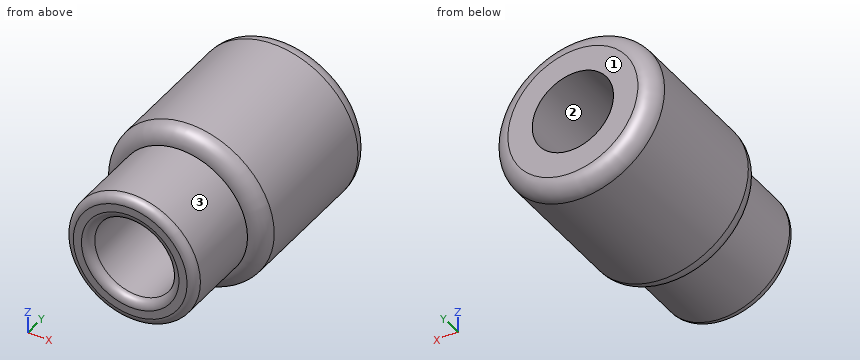
```python
from build123d import *

# Parameters (mm, degrees)
F0_R     = 127
F1_DEPTH = 254
F2_R     = 25.4
F4_D     = 127
F5_DEPTH = 127
F6_R     = 12.7


# Not quite as in the source:
# - a feature names something its author has since deleted; it is built from what else it names


with BuildPart() as f1:
    # F0 (on Front) → F1 (new body)
    with BuildSketch(Plane.XZ):
        Circle(F0_R)
    extrude(amount=F1_DEPTH)

    # F2
    f2_edges = [f1.edges().sort_by_distance(p)[0] for p in [
        (-127, -254, 0),
        (-127, 0, 0),
    ]]
    fillet(f2_edges, radius=F2_R)

    # F4 (through all)
    with Locations(Plane.XZ.offset(254)):
        with Locations((0, 0)):
            Hole(F4_D / 2)

    # F5 (add): a face of the model
    f5_faces = [f1.faces().sort_by_distance(p)[0] for p in [
        (-98.7263180413, -254, 0),
    ]]
    extrude(f5_faces, amount=F5_DEPTH)

    # F6
    f6_edges = [f1.edges().sort_by_distance(p)[0] for p in [
        (-101.6, -381, 0),
        (-63.5, -381, 0),
    ]]
    fillet(f6_edges, radius=F6_R)


solid = f1.part
```
Model file for the job. Use its own axes, mm. Face numbers are marked on the shaded views. Coordinates: 2 decimals unless noted, no trailing zeros. Order: outer loops, then holes, each group sorted by start corner. A loop starts at its lowest first (then second) coordinate and runs counter-clockwise, first axis right, second up. Notation, with made-up numbers: (42, 68) -> (80, 68) arc R17 ccw to (80, 79) -> close; hole circle Ø5 at (11, 67.5). An arc over 180 degrees is marked (long way). Answer as a JSON object with one key per item and string values. Group by question number.
1) Flat gauge pins, fed straight in: pin 1 (2 mm diameter, centred on y = -223.5, z = 40.5, fed in from -X); pin 2 (8 mm diameter, centred on x = -94.5, y = -201.5, fed in from +Z); pin 3 (1 mm diameter, centred on x = -45, y = -309.5, fed in from +Z). Where does each tip first touch, or does it go through?
2) Cut at A-A, the plane x = 0. Write the cut outline in (y, z).
3) Cut at B-B, the plane z = 0. Write the cut outline in (x, y).
4) Pull direction Z, two halves, no side cores. Call the marked faces 1, 2 and 3: +Z half, -Z half, draft (parallel to the pull), parting line (faces both ways), or undercut.
5) Cut at C-C, the plane y = -205. Write the cut outline in (x, z).
6) Drill centre lines: L1, parallel to Z at x = 0, y = -214; L2, parallel to Z at x = 0, y = -288; L3, parallel to X at y = -274, z = 22. Where is each one in solid material? Low to high.
Check values:
{
 "1": {"pin 1": "stops at x = -120.7", "pin 2": "stops at z = 89.1", "pin 3": "stops at z = 91.34"},
 "2": {"outline": "(-381, -88.9) arc R12.7 ccw to (-368.3, -101.6) -> (-254, -101.6) arc R25.4 ccw to (-228.6, -127) -> (-25.4, -127) arc R25.4 ccw to (0, -101.6) -> (0, -63.5) -> (-368.3, -63.5) arc R12.7 ccw to (-381, -76.2) -> close; (-381, 76.2) arc R12.7 ccw to (-368.3, 63.5) -> (0, 63.5) -> (0, 101.6) arc R25.4 ccw to (-25.4, 127) -> (-228.6, 127) arc R25.4 ccw to (-254, 101.6) -> (-368.3, 101.6) arc R12.7 ccw to (-381, 88.9) -> close"},
 "3": {"outline": "(-127, -228.6) arc R25.4 ccw to (-101.6, -254) -> (-101.6, -368.3) arc R12.7 ccw to (-88.9, -381) -> (-76.2, -381) arc R12.7 ccw to (-63.5, -368.3) -> (-63.5, 0) -> (-101.6, 0) arc R25.4 ccw to (-127, -25.4) -> close; (63.5, -368.3) arc R12.7 ccw to (76.2, -381) -> (88.9, -381) arc R12.7 ccw to (101.6, -368.3) -> (101.6, -254) arc R25.4 ccw to (127, -228.6) -> (127, -25.4) arc R25.4 ccw to (101.6, 0) -> (63.5, 0) -> close"},
 "4": {"face 1": "draft", "face 2": "undercut", "face 3": "parting line"},
 "5": {"outline": "circle Ø254 at (0, 0); hole circle Ø127 at (0, 0)"},
 "6": {"L1": "z = -127 to -63.5, 63.5 to 127", "L2": "z = -101.6 to -63.5, 63.5 to 101.6", "L3": "x = -99.19 to -59.57, 59.57 to 99.19"}
}
